The drawing under review shows one solid part. Ordinate dimensions are in mm from its lowest x, y, z. Coordinates: 2 decimals unless noted, no trailing zeros. Write each loop counter-clockwise with the first axis right and the second up, starting at its lowest first coordinate (ties: lowest second). Pieces come first, ordered by that corner, then holes.
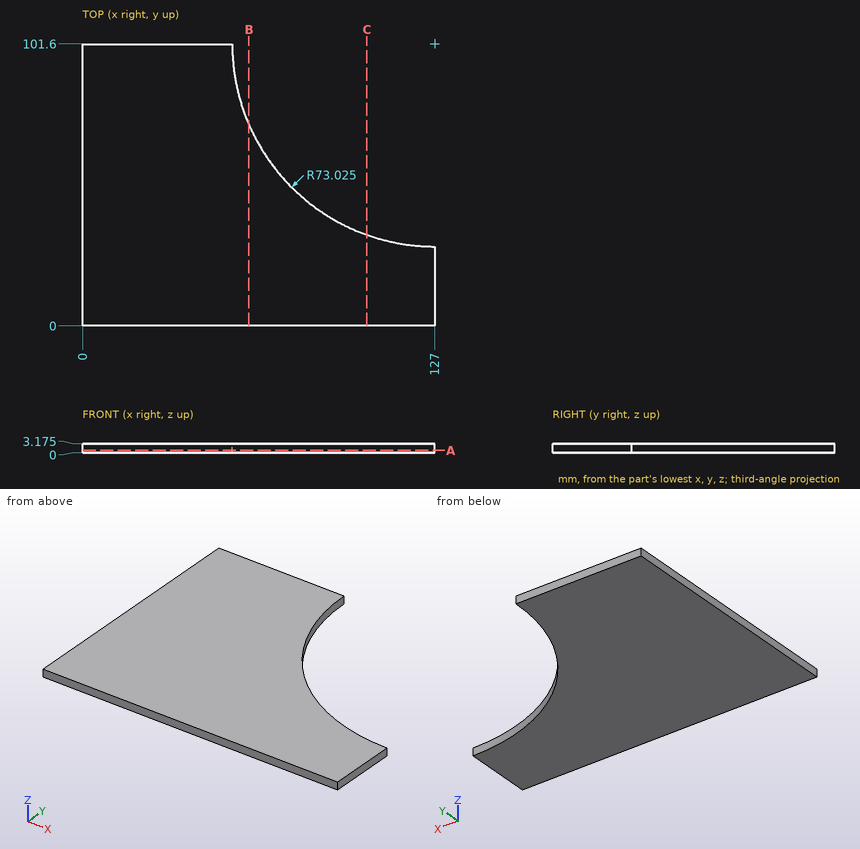
Q1. Add section B-B (x = 60). State the section outline as (y, z) points (3 decimals), then the cut area to 3 significant figures.
Ans:
outline: (0, 0) - (72.554, 0) - (72.554, 3.175) - (0, 3.175) - close
area: 230 mm2
Q2. Add section C-C (x = 102.5). State the section outline as (y, z) points (3 decimals).
Ans:
outline: (0, 0) - (32.808, 0) - (32.808, 3.175) - (0, 3.175) - close
Q3. For probe 1 along X at (y, z) = (66, 1.45); probe 2 along X at (y, z) = (47, 0.2); probe 3 along Y at (x, z) = (68, 1), list the stretches that pass through material, from the lowest coordinate up.
Ans:
probe 1: x = 0 to 63.24
probe 2: x = 0 to 78.51
probe 3: y = 0 to 58.57
Q4. Add section A-A (z = 0.8). State the section outline as (x, y) points (3 decimals), then the cut area to 3 significant figures.
Ans:
outline: (0, 0) - (127, 0) - (127, 28.575) arc R73.025 cw to (53.975, 101.6) - (0, 101.6) - close
area: 8,710 mm2
